Answer from the drawing. Dimensions are ordinates in mm from the lowest x, y and z of the part. A direction names the side the tool comes from. Round coordinates to 2 decimals unless told otherwise and drop trailing zeros. Order: outer loops, then holes, each group sorted by start corner. A loop starts at its lowest first (then second) coordinate and runs counter-clockwise, first axis right, second up.
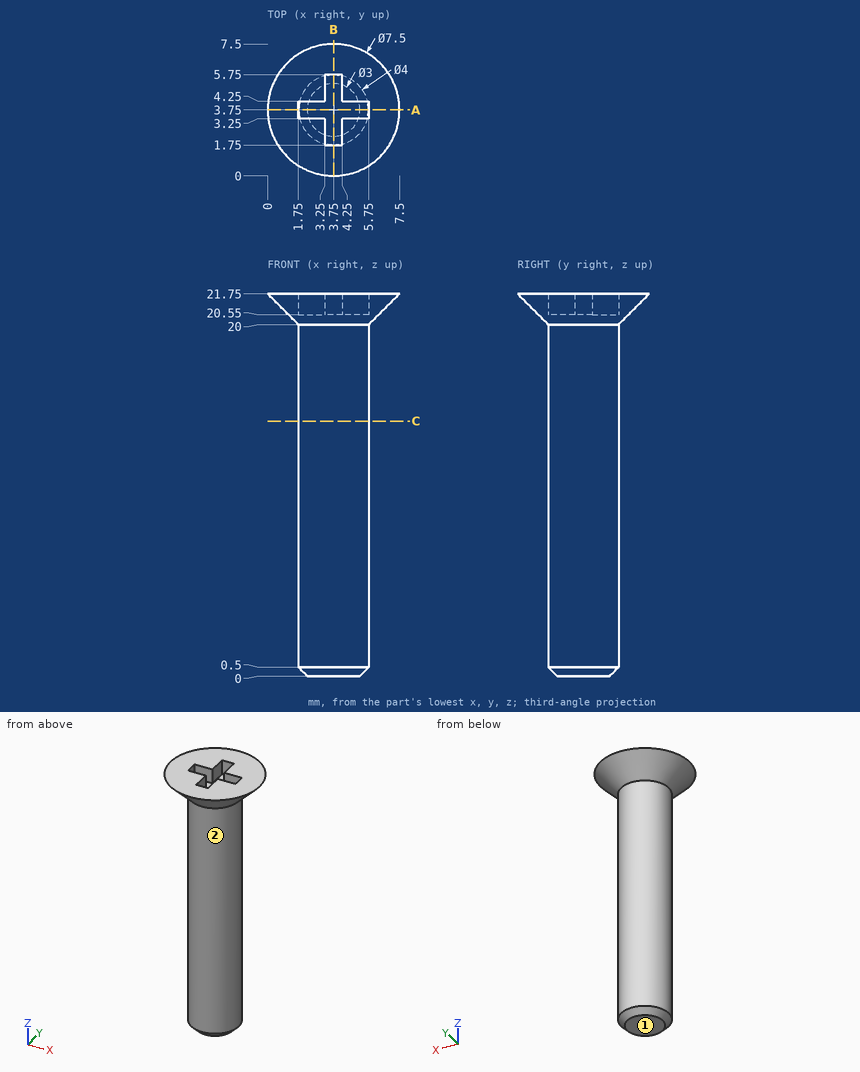
Q1. Flat-ended cylindrical pins translate along their axes: pin 1 (1.2 mm diameter, centred on x = 4.5, y = 3.5, fed in from +Z); pin 2 (1 mm diameter, centred on x = 3.5, z = 11, fed in from +Y); pin 3 (1.1 mm diameter, centred on y = 3.5, z = 21, fed in from -X); pin 4 (1.3 mm diameter, centred on x = 5, z = 21.5, fed in from -Y). Find the tip coordinate at first contact, or state that the pin passes through.
Outcome:
pin 1: stops at z = 21.75
pin 2: stops at y = 5.75
pin 3: stops at x = 0.21
pin 4: stops at y = 0.06
Q2. A cutting plane is placed at C-C, the plane z = 14.5. Give the vertices of the cut face in (x, y).
Outcome:
outline: circle Ø4 at (3.75, 3.75)
Q3. Straight lines are drawn through the part: probe 1 along Z at (x, y) = (4, 2.5); probe 2 along X at (y, z) = (5.5, 9.5); probe 3 along X at (y, z) = (2.5, 13.5). For each, find the intervals that lie inside material, in ascending order.
Outcome:
probe 1: z = 0 to 20.55
probe 2: x = 2.78 to 4.72
probe 3: x = 2.19 to 5.31
Q4. A cutting plane is placed at A-A, the plane y = 3.75. Give the vertices of the cut face in (x, z), plus the area to 3 significant figures.
Outcome:
outline: (0, 21.75) - (1.75, 20) - (1.75, 0.5) - (2.25, 0) - (5.25, 0) - (5.75, 0.5) - (5.75, 20) - (7.5, 21.75) - (5.75, 21.75) - (5.75, 20.55) - (1.75, 20.55) - (1.75, 21.75) - close
area: 85.0 mm2
Q5. For the marked faces 1 and 2, determine the directions among +Z, -Z, +X, -X, +Y, -Y from which every point of the face is accessible in a straight line to the end or side of a thin tool.
Outcome:
face 1: -Z, +X, -X, +Y, -Y
face 2: -Z
